For this review, use the dimensioned drawing (mm, ordinates from the lowest corner) and the shaded views. A direction names the side the tool comes from. Round coordinates to 2 decimals unless told otherwise and drop trailing zeros. Write each loop counter-clockwise with the first axis right and the second up, starting at its lowest first coordinate (ties: lowest second). Pieces come first, ordered by that corner, then holes.
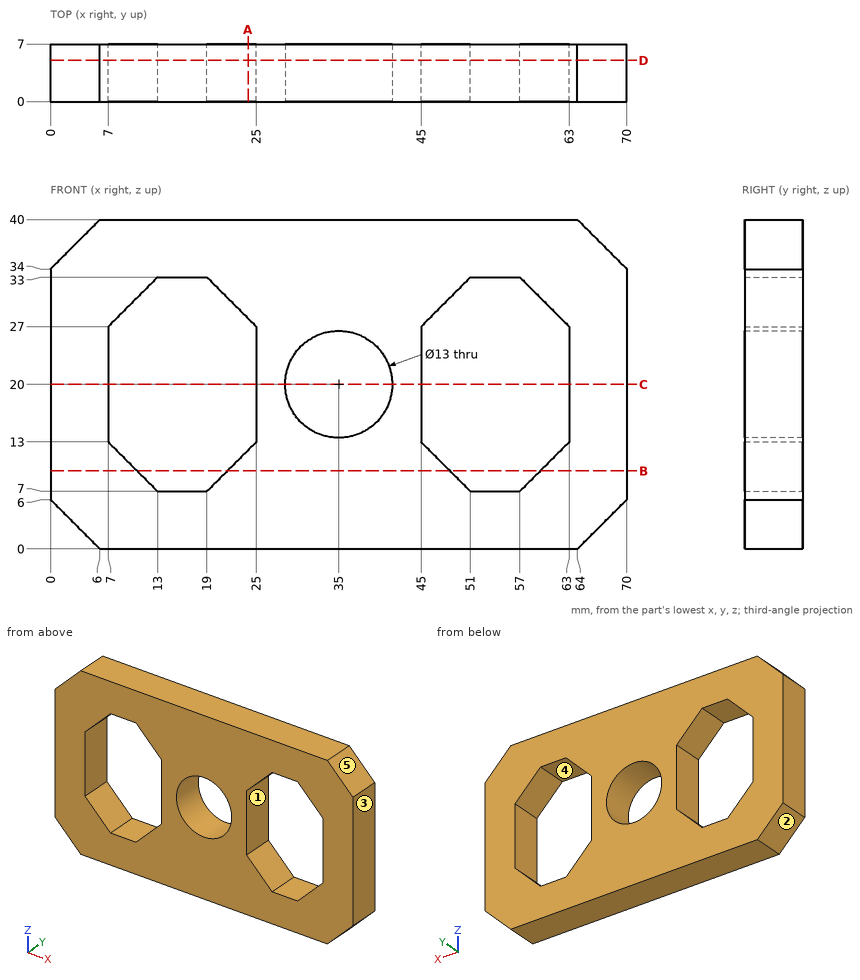
1) For P1, Ø5, axis at x = 36, z = 22.5, coming from the +Y side, flat-tipped, find the tip position at first contact; note if it passes through.
2) Add section C-C on z = 20. State the section outline as (x, y) points.
3) Add section D-D on y = 5. State the section outline as (x, z) points.
4) For the marked faces 4 and 5, list the 3-axis set-ups (+Z, -Z, +X, -X, +Y, -Y) from which the entire face can be reached by the end or side of a thin tool; tool diameter is ignored.
5) Add section B-B on z = 9.5. State the section outline as (x, y) points.
6) For line 1 along X through (y, z) = (4, 20); line 2 along X through (y, z) = (0.75, 30.5); line 3 along X through (y, z) = (2.5, 32), list the stretches that pass through material, from the lowest coordinate up.
7) Add section A-A on x = 24. State the section outline as (y, z) points, and give its area (3 significant figures).
8) The part is to be moulded in two halves that separate along X. For the marked faces 1, 2 and 3, say which applies: pulls with the +X half, pulls with the -X half, needs draft (parallel to the pull), parting line crosses it, or undercut.
Computed:
1. P1: passes through
2. outline: (0, 0) - (7, 0) - (7, 7) - (0, 7) - close; (25, 0) - (28.5, 0) - (28.5, 7) - (25, 7) - close; (41.5, 0) - (45, 0) - (45, 7) - (41.5, 7) - close; (63, 0) - (70, 0) - (70, 7) - (63, 7) - close
3. outline: (0, 6) - (6, 0) - (64, 0) - (70, 6) - (70, 34) - (64, 40) - (6, 40) - (0, 34) - close; hole (7, 13) - (13, 7) - (19, 7) - (25, 13) - (25, 27) - (19, 33) - (13, 33) - (7, 27) - close; hole circle Ø13 at (35, 20); hole (45, 13) - (51, 7) - (57, 7) - (63, 13) - (63, 27) - (57, 33) - (51, 33) - (45, 27) - close
4. face 4: +Y, -Y
4. face 5: +Z, +X, +Y, -Y
5. outline: (0, 0) - (10.5, 0) - (10.5, 7) - (0, 7) - close; (21.5, 0) - (48.5, 0) - (48.5, 7) - (21.5, 7) - close; (59.5, 0) - (70, 0) - (70, 7) - (59.5, 7) - close
6. line 1: x = 0 to 7, 25 to 28.5, 41.5 to 45, 63 to 70
6. line 2: x = 0 to 10.5, 21.5 to 48.5, 59.5 to 70
6. line 3: x = 0 to 12, 20 to 50, 58 to 70
7. outline: (0, 0) - (7, 0) - (7, 12) - (0, 12) - close; (0, 28) - (7, 28) - (7, 40) - (0, 40) - close
7. area: 168 mm2
8. face 1: undercut
8. face 2: pulls with the -X half
8. face 3: pulls with the +X half
